```python
from build123d import *

# Parameters (mm, degrees)
F1_ANGLE = 180


with BuildPart() as f1:
    # F0 (on Top) → F1 (revolve)
    with BuildSketch(Plane.XY):
        with BuildLine():
            Line((-50.8, -101.6), (-46.288617, -101.6))
            Line((-46.288617, -101.6), (-46.288617, 101.09959))
            ThreePointArc((-46.288617, 101.09959), (-46.291322, 101.6), (-46.288617, 102.10041))
            ThreePointArc((-46.288617, 102.10041), (-32.555505, 134.509353), (0, 147.891322))
            Line((0, 147.891322), (0, 152.4))
            ThreePointArc((0, 152.4), (-35.921024, 137.521024), (-50.8, 101.6))
            Line((-50.8, 101.6), (-50.8, -101.6))
        make_face()
    revolve(axis=Axis((0, 0, 0), (0, -1, 0)), revolution_arc=F1_ANGLE)


solid = f1.part
```
Geometry check sheet. Reference: the model listing, model coordinates, mm. Round coordinates to 2 decimals unless told otherwise and drop trailing zeros. Write each question's results on one line, items separated by ' | '.
(1) Thickness scan on probe 1 along X at (y, z) = (44, -38); probe 2 along X at (y, z) = (111, -28); probe 3 along Z at (x, y) = (42, 24.5). Record the ranges inside material, lowest first. Write a range as from..to.
Computed:
probe 1: x = -33.71..-26.43, 26.43..33.71 | probe 2: x = -41.33..-35.64, 35.64..41.33 | probe 3: z = -28.58..-19.46
(2) Depth check by flat-ended pin: pin 1 Ø5 at (y, z) = (-42.5, -22.5) entering from -X; pin 2 Ø4 at (x, y) = (9.5, 73.5) entering from +Z; pin 3 Ø3 at (y, z) = (108, -45.5) entering from +X; pin 4 Ø10 at (x, z) = (37.5, -45) entering from -Y. Enter the tip coordinate at first touch or a pass-through.
Computed:
pin 1: stops at x = -46.7 | pin 2: stops at z = -44.84 | pin 3: stops at x = 24.6 | pin 4: passes through
(3) Draft check along X on faces 1 (the face through (-7, -101.6, -46)), 2 (the face through (-1.117, -1.422, -50.788)), 3 (the face through (-1.018, 1.169, -46.277)). Enter one of: pulls with the +X half, pulls with the -X half, needs draft (parallel to the pull), parting line crosses it, or undercut.
Computed:
face 1: needs draft | face 2: parting line crosses it | face 3: undercut
